```python
from build123d import *

# Parameters (mm, degrees)
SKETCH1_R           = 450
BOSS_EXTRUDE1_DEPTH = 10
SKETCH2_R           = 70
BOSS_EXTRUDE2_DEPTH = 40
BOSS_EXTRUDE3_DEPTH = 10


with BuildPart() as part:
    # Sketch1 → Boss-Extrude1 (new body)
    with BuildSketch(Plane.XY):
        Circle(SKETCH1_R)
        with BuildLine():
            Line((28.284271247, -10), (50, -10))
            Line((50, -10), (50, 10))
            Line((50, 10), (28.284271247, 10))
            ThreePointArc((28.284271247, 10), (0, 30), (-28.284271247, 10))
            Line((-28.284271247, 10), (-50, 10))
            Line((-50, 10), (-50, -10))
            Line((-50, -10), (-28.284271247, -10))
            ThreePointArc((-28.284271247, -10), (0, -30), (28.284271247, -10))
        make_face(mode=Mode.SUBTRACT)
    extrude(amount=BOSS_EXTRUDE1_DEPTH)

    # Sketch2 → Boss-Extrude2 (add)
    with BuildSketch(Plane.XY.offset(10)):
        Circle(SKETCH2_R)
        with BuildLine():
            Line((-50, 10), (-50, -10))
            Line((-50, -10), (-28.284271247, -10))
            ThreePointArc((-28.284271247, -10), (0, -30), (28.284271247, -10))
            Line((28.284271247, -10), (50, -10))
            Line((50, -10), (50, 10))
            Line((50, 10), (28.284271247, 10))
            ThreePointArc((28.284271247, 10), (0, 30), (-28.284271247, 10))
            Line((-28.284271247, 10), (-50, 10))
        make_face(mode=Mode.SUBTRACT)
    extrude(amount=BOSS_EXTRUDE2_DEPTH)

    # Sketch3 → Boss-Extrude3 (add)
    with BuildSketch(Plane.XY.offset(10)):
        with BuildLine():
            Line((-47.935658511, 547.90708395), (-34.862297099, 398.477879237))
            ThreePointArc((-34.862297099, 398.477879237), (-17.447754946, 399.619288633), (0, 400))
            ThreePointArc((0, 400), (17.447754946, 399.619288633), (34.862297099, 398.477879237))
            Line((34.862297099, 398.477879237), (47.935658511, 547.90708395))
            ThreePointArc((47.935658511, 547.90708395), (0, 550), (-47.935658511, 547.90708395))
        make_face()
        with BuildLine():
            Line((450.533624359, 315.467039993), (327.660817716, 229.43057454))
            ThreePointArc((327.660817716, 229.43057454), (346.410161514, 200), (362.523114815, 169.047304696))
            Line((362.523114815, 169.047304696), (498.46928287, 232.440043957))
            ThreePointArc((498.46928287, 232.440043957), (476.313972081, 275), (450.533624359, 315.467039993))
        make_face()
        with BuildLine():
            Line((498.46928287, -232.440043957), (362.523114815, -169.047304696))
            ThreePointArc((362.523114815, -169.047304696), (346.410161514, -200), (327.660817716, -229.43057454))
            Line((327.660817716, -229.43057454), (450.533624359, -315.467039993))
            ThreePointArc((450.533624359, -315.467039993), (476.313972081, -275), (498.46928287, -232.440043957))
        make_face()
        with BuildLine():
            Line((47.935658511, -547.90708395), (34.862297099, -398.477879237))
            ThreePointArc((34.862297099, -398.477879237), (0, -400), (-34.862297099, -398.477879237))
            Line((-34.862297099, -398.477879237), (-47.935658511, -547.90708395))
            ThreePointArc((-47.935658511, -547.90708395), (0, -550), (47.935658511, -547.90708395))
        make_face()
        with BuildLine():
            Line((-450.533624359, -315.467039993), (-327.660817716, -229.43057454))
            ThreePointArc((-327.660817716, -229.43057454), (-346.410161514, -200), (-362.523114815, -169.047304696))
            Line((-362.523114815, -169.047304696), (-498.46928287, -232.440043957))
            ThreePointArc((-498.46928287, -232.440043957), (-476.313972081, -275), (-450.533624359, -315.467039993))
        make_face()
        with BuildLine():
            Line((-498.46928287, 232.440043957), (-362.523114815, 169.047304696))
            ThreePointArc((-362.523114815, 169.047304696), (-346.410161514, 200), (-327.660817716, 229.43057454))
            Line((-327.660817716, 229.43057454), (-450.533624359, 315.467039993))
            ThreePointArc((-450.533624359, 315.467039993), (-476.313972081, 275), (-498.46928287, 232.440043957))
        make_face()
    extrude(amount=-BOSS_EXTRUDE3_DEPTH)


solid = part.part
```
Check sheet for the modelled part. Datum: model origin and axes. Units: mm. A direction names the side the tool comes from. Round coordinates to 2 decimals unless told otherwise and drop trailing zeros. Loops run counter-clockwise (first coordinate to the right, second up) from the corner with the lowest first, then second, coordinate; pieces in that order, holes last. Notation, with made-up numbers: (38.5, -8) - (96.5, -8) arc R28 cw to (96.5, 31) - close; hole circle Ø1 at (32.5, 86). An arc over 180 degrees is marked (long way). Write item = value, one per line. Start each with the question number.
Q1. Depth check by flat-ended pin: P1, Ø22, axis at y = -2, z = 33.5, coming from the -X side; P2, Ø10, axis at x = -371.5, y = -141.5, coming from the +Z side; P3, Ø6.5, axis at x = -35.5, z = 33.5, coming from the -Y side. Enter the tip coordinate at first touch or a pass-through.
Q2. Access from +Z, -Z, +X, -X, +Y, -Y to the whole of each face (thin tool, end or side, straight path). Record for faces 4 (the face through (452.519, 211.013, 5.07)), 5 (the face through (476.65, 274.42, 5.07)), 6 (the face through (104, 8, 0)), 7 (the face through (-410.15, -287.19, 5.07)), 8 (the face through (-452.519, -211.013, 5.07)).
Q3. Section check C-C (y = -353). Record the boundary of the cut face in (x, z), plus the area to 3 significant figures.
Q4. Section check B-B (z = 34). Record the boundary of the cut face in (x, y).
Q5. Section check A-A (x = 0). Record the boundary of the cut face in (y, z), plus the area to 3 significant figures.
Q6. Release check for a two-part mould opening along X. For faces 1 (the face through (-55.55, -42.594, 29.72)), 2 (the face through (449.99, -2.75, 4.93)), 3 (the face through (410.15, 287.19, 5.07)) record: pulls with the +X half, pulls with the -X half, needs draft (parallel to the pull), parting line crosses it, or undercut.
Q7. Thickness scan on L1, parallel to Z at x = 96.5, y = -252; L2, parallel to Y at x = -7, z = 2.5; L3, parallel to Y at x = -1, z = 19. Record the ranges inside material, lowest first.
Q8. Section check D-D (x = -147). Record the boundary of the cut face in (y, z).
Derived:
q1.P1 = -70
q1.P2 = 10
q1.P3 = -62.13
q2.face_4 = +Z, -Z, +X
q2.face_5 = +Z, -Z, +X, +Y
q2.face_6 = -Z, +X, -X, +Y, -Y
q2.face_7 = +Z, -Z, -Y
q2.face_8 = +Z, -Z, -X
q3.outline = (-279.09, 0) - (279.09, 0) - (279.09, 10) - (-279.09, 10) - close
q3.area = 5,580 mm^2
q4.outline = circle Ø140 at (0, 0); hole (-50, -10) - (-28.28, -10) arc R30 ccw to (28.28, -10) - (50, -10) - (50, 10) - (28.28, 10) arc R30 ccw to (-28.28, 10) - (-50, 10) - close
q5.outline = (-550, 0) - (-30, 0) - (-30, 50) - (-70, 50) - (-70, 10) - (-550, 10) - close; (30, 0) - (550, 0) - (550, 10) - (70, 10) - (70, 50) - (30, 50) - close
q5.area = 13,600 mm^2
q6.face_1 = parting line crosses it
q6.face_2 = pulls with the +X half
q6.face_3 = undercut
q7.L1 = 0 to 10
q7.L2 = -549.96 to -29.17, 29.17 to 549.96
q7.L3 = -69.99 to -29.98, 29.98 to 69.99
q8.outline = (-425.31, 0) - (425.31, 0) - (425.31, 10) - (-425.31, 10) - close
